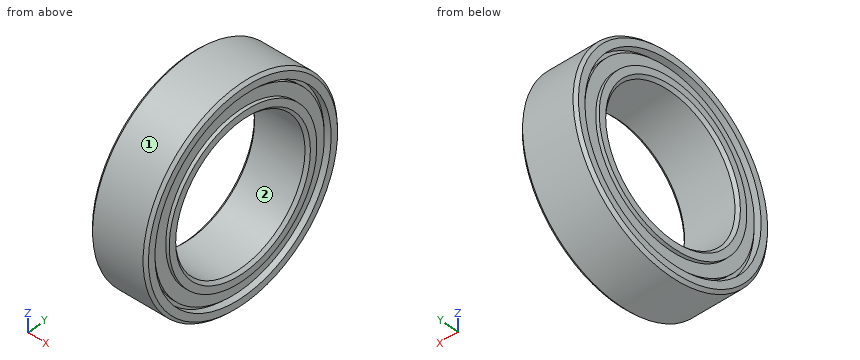
from build123d import *

# Parameters (mm, degrees)
CHAMFER_1_SIZE = 0.2


with BuildPart() as part:
    # 草图1 → 旋转1 (revolve)
    with BuildSketch(Plane.XY, mode=Mode.PRIVATE) as revolve_1_sk:
        Polygon((-2, 5), (2, 5), (2, 5.7), (1.75, 5.7), (1.75, 6.55), (1.5, 6.55), (1.5, 6.8), (2, 6.8), (2, 7.5), (-2, 7.5), (-2, 6.8), (-1.5, 6.8), (-1.5, 6.55), (-1.75, 6.55), (-1.75, 5.7), (-2, 5.7), align=None)
    revolve(revolve_1_sk.sketch.rotate(Axis((-3.90102381, 0, 0), (1, 0, 0)), 90), axis=Axis((-3.90102381, 0, 0), (1, 0, 0)))

    # 倒角1
    chamfer_1_edges = [part.edges().sort_by_distance(p)[0] for p in [
        (-2, 0, -7.5),
        (2, 0, -7.5),
        (2, 0, -5),
        (-2, 0, -5),
    ]]
    chamfer(chamfer_1_edges, length=CHAMFER_1_SIZE)


solid = part.part
Could you check a few things on this model? Use its own coordinates, in mm. Face numbers are marked on the shaded views. Coordinates: 2 decimals unless noted, no trailing zeros. Order: outer loops, then holes, each group sorted by start corner. A loop starts at its lowest first (then second) coordinate and runs counter-clockwise, first axis right, second up.
Q1. Thinking about a two-plate mould opening in Y: for the marked faces 1 and 2, which applies, released by +Y, released by -Y, zero draft, split by the parting line, or undercut?
Q2. Will these pins go through, and if not, where does the flat tip stop? pin 1 (9 mm diameter, centred on y = 0, z = 0, fed in from -X); pin 2 (2 mm diameter, centred on x = 0, z = -1.5, fed in from -Y).
Q3. Suppose I cut it at A-A on x = -0.35. Please give me the cut outline in (y, z).
Q4. Please list where these lines run through material, in increasing order: L1, parallel to Y at x = 1.65, z = 0; L2, parallel to Y at x = 1.85, z = 0; L3, parallel to Z at x = 1.2, y = 4.
Answer:
1. face 1: split by the parting line
1. face 2: undercut
2. pin 1: passes through
2. pin 2: stops at y = -7.48
3. outline: circle Ø15 at (0, 0); hole circle Ø10 at (0, 0)
4. L1: y = -7.5 to -6.8, -6.55 to -5, 5 to 6.55, 6.8 to 7.5
4. L2: y = -7.45 to -6.8, -5.7 to -5.05, 5.05 to 5.7, 6.8 to 7.45
4. L3: z = -6.34 to -3, 3 to 6.34
